```python
from build123d import *

# Parameters (mm, degrees)
F0_R     = 4.2545
F0_R_2   = 41.275
F1_DEPTH = 38.1
F2_R     = 8.001
F2_R_2   = 4.2545
F3_DEPTH = 6.35
F2_R_3   = 47.625
F2_R_4   = 44.45
F4_DEPTH = 3.175


with BuildPart() as f1:
    # F0 (on Top) → F1 (new body)
    with BuildSketch(Plane.XY):
        with BuildLine():
            Line((64.06365, -25.199729), (60.788761, 18.400254))
            ThreePointArc((60.788761, 18.400254), (0, 74.794278), (-60.788761, 18.400254))
            Line((-60.788761, 18.400254), (-64.06365, -25.199729))
            ThreePointArc((-64.06365, -25.199729), (-60.533997, -40.139233), (-49.042173, -50.316916))
            ThreePointArc((-49.042173, -50.316916), (0, -60.714722), (49.042173, -50.316916))
            ThreePointArc((49.042173, -50.316916), (60.533997, -40.139233), (64.06365, -25.199729))
        make_face()
        with Locations((-49.276, -34.477577)):
            Circle(F0_R, mode=Mode.SUBTRACT)
        with Locations((49.276, -34.477577)):
            Circle(F0_R, mode=Mode.SUBTRACT)
        Circle(F0_R_2, mode=Mode.SUBTRACT)
        with Locations((0, 60.140065)):
            Circle(F0_R, mode=Mode.SUBTRACT)
    extrude(amount=F1_DEPTH)

    # F2 (on face) → F3 (cut)
    with BuildSketch(Plane.XY.offset(38.1)):
        with Locations((0, 60.140065)):
            Circle(F2_R)
        with Locations((0, 60.140065)):
            Circle(F2_R_2, mode=Mode.SUBTRACT)
        with Locations((-49.276, -34.477577)):
            Circle(F2_R)
        with Locations((-49.276, -34.477577)):
            Circle(F2_R_2, mode=Mode.SUBTRACT)
        with Locations((49.276, -34.477577)):
            Circle(F2_R)
        with Locations((49.276, -34.477577)):
            Circle(F2_R_2, mode=Mode.SUBTRACT)
    extrude(amount=-F3_DEPTH, mode=Mode.SUBTRACT)

    # F2 (on face) → F4 (cut)
    with BuildSketch(Plane.XY.offset(38.1)):
        Circle(F2_R_3)
        Circle(F2_R_4, mode=Mode.SUBTRACT)
    extrude(amount=-F4_DEPTH, mode=Mode.SUBTRACT)


solid = f1.part
```
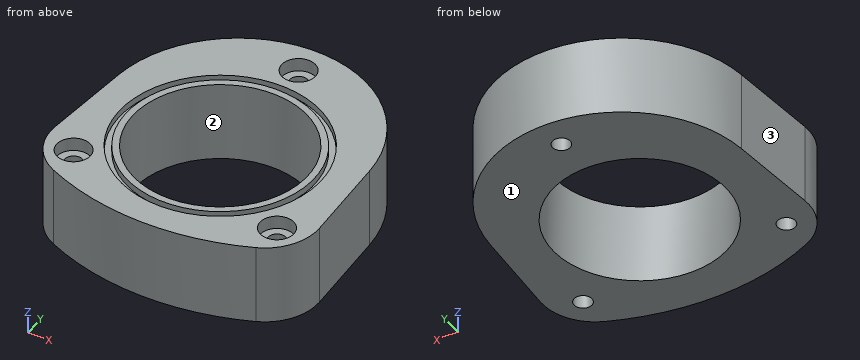
Model file for the job. Use its own axes, mm. Face numbers are marked on the shaded views. Round coordinates to 2 decimals unless told otherwise and drop trailing zeros. Order: outer loops, then holes, each group sorted by start corner. A loop starts at its lowest first (then second) coordinate and runs counter-clockwise, first axis right, second up. Notation, with made-up numbers: (-9.75, -38) -> (-4.75, -38) arc R32 ccw to (-4.75, -6) -> close; hole circle Ø4 at (78, 62). An arc over 180 degrees is marked (long way). Use one line per item in the form item = value.
Item 1: Cut at B-B, the plane y = -19.5. Write the cut outline in (x, z) (3 decimals).
Returned:
outline = (-63.636, 0) -> (-36.378, 0) -> (-36.378, 38.1) -> (-39.944, 38.1) -> (-39.944, 34.925) -> (-43.45, 34.925) -> (-43.45, 38.1) -> (-63.636, 38.1) -> close; (36.378, 0) -> (63.636, 0) -> (63.636, 38.1) -> (43.45, 38.1) -> (43.45, 34.925) -> (39.944, 34.925) -> (39.944, 38.1) -> (36.378, 38.1) -> close
Item 2: Cut at C-C, the plane x = -27. Write the cut outline in (y, z) (3 decimals).
Returned:
outline = (-57.66, 0) -> (-31.219, 0) -> (-31.219, 38.1) -> (-35.31, 38.1) -> (-35.31, 34.925) -> (-39.232, 34.925) -> (-39.232, 38.1) -> (-57.66, 38.1) -> close; (31.219, 0) -> (68.489, 0) -> (68.489, 38.1) -> (39.232, 38.1) -> (39.232, 34.925) -> (35.31, 34.925) -> (35.31, 38.1) -> (31.219, 38.1) -> close
Item 3: Drill centre lines: line 1 (Y direction, x = 0, z = 35) (3 decimals); line 2 (X direction, y = -35, z = 9); line 3 (Z direction, x = 45, y = -38). Where is each one in solid material? Low to high.
Returned:
line_1 = -60.715 to -47.625, -44.45 to -41.275, 41.275 to 44.45, 47.625 to 52.139, 68.141 to 74.794
line_2 = -62.88 to -53.5, -45.05 to -21.88, 21.88 to 45.05, 53.5 to 62.88
line_3 = 0 to 31.75
Item 4: Cut at D-D, the plane z = 29.5. Give the number of separate pieces and of enclosed holes in the cut face, and give its area (3 significant figures).
Returned:
separate_pieces = 1
enclosed_holes = 4
area = 8,910 mm^2
Item 5: Pull direction Y, two halves, no side cores. Call the marked faces 1, 2 and 3: released by +Y, released by -Y, zero draft, split by the parting line, or undercut.
Returned:
face_1 = zero draft
face_2 = undercut
face_3 = released by +Y
Item 6: Cut at A-A, the plane x = 0. Write the cut outline in (y, z) (3 decimals), and give its area (3 significant figures).
Returned:
outline = (-60.715, 0) -> (-41.275, 0) -> (-41.275, 38.1) -> (-44.45, 38.1) -> (-44.45, 34.925) -> (-47.625, 34.925) -> (-47.625, 38.1) -> (-60.715, 38.1) -> close; (41.275, 0) -> (55.886, 0) -> (55.886, 31.75) -> (52.139, 31.75) -> (52.139, 38.1) -> (47.625, 38.1) -> (47.625, 34.925) -> (44.45, 34.925) -> (44.45, 38.1) -> (41.275, 38.1) -> close; (64.395, 0) -> (74.794, 0) -> (74.794, 38.1) -> (68.141, 38.1) -> (68.141, 31.75) -> (64.395, 31.75) -> close
area = 1,630 mm^2
Item 7: Flat gauge pins, fed straight in: pin 1 Ø10 at (x, z) = (30, 26) entering from +Y; pin 2 Ø2 at (x, z) = (39.5, 12.5) entering from +Y; pin 3 Ø7.5 at (x, y) = (0, 60.14) entering from -Z; pin 4 Ø11 at (x, y) = (-49.28, -34.48) entering from +Z. Where does each tip first touch, or does it go through?
Returned:
pin_1 = 69.43
pin_2 = 61.1
pin_3 = through
pin_4 = 31.75
